Source: CAD feature listing. Evaluate the final solid. Frame: model axes, mm. Face numbers are marked on the shaded views. A direction names the side the tool comes from. Coordinates: 2 decimals unless noted, no trailing zeros. Order: outer loops, then holes, each group sorted by start corner. A loop starts at its lowest first (then second) coordinate and runs counter-clockwise, first axis right, second up.
Autodesk Inventor part; units mm, degrees
ref_plane "YZ Plane" through (0, 0, 0) normal (1, 0, 0) x (0, 1, 0)
ref_plane "XZ Plane" through (0, 0, 0) normal (0, 1, 0) x (-1, 0, 0)
ref_plane "XY Plane" through (0, 0, 0) normal (0, 0, 1) x (1, 0, 0)
sketch "Sketch1" plane through (0, 0, 0) normal (0, 1, 0) x (-1, 0, 0)
  line L0 (35, -17.5) -> (-35, -17.5)
  line L1 (-35, -17.5) -> (-35, 17.5)
  line L2 (-35, 17.5) -> (35, 17.5)
  line L3 (35, 17.5) -> (35, -17.5)
  line L4 (35, -17.5) -> (-35, 17.5) construction
  line L5 (-35, -17.5) -> (35, 17.5) construction
  point P0 (0, 0)
  dimension "d0" = 70
  dimension "d1" = 35
extrude "Extrusion1" add sketch "Sketch1" along normal blind 19.05
sketch "Sketch2" plane through (0, 19.05, 0) normal (0, 1, 0) x (1, 0, 0)
  line L0 (32.5, -15) -> (-32.5, -15)
  line L1 (-32.5, -15) -> (-32.5, 15)
  line L2 (-32.5, 15) -> (32.5, 15)
  line L3 (32.5, 15) -> (32.5, -15)
  line L4 (32.5, -15) -> (-32.5, 15) construction
  line L5 (-32.5, -15) -> (32.5, 15) construction
  point P0 (0, 0)
  dimension "d4" = 65
  dimension "d5" = 30
extrude "Extrusion2" cut sketch "Sketch2" against normal blind 1.5875
fillet "Fillet1" radius 3 4 edges at (-32.5, 18.2563, -15) (-32.5, 18.2563, 15) (32.5, 18.2563, -15) (32.5, 18.2563, 15)
sketch "Sketch3" plane through (0, 17.4625, 0) normal (0, 1, 0) x (1, 0, 0)
  arc A0 (-29.5, 15) -> (-32.5, 12) centre (-29.5, 12) ccw
  arc A1 (-32.5, -12) -> (-29.5, -15) centre (-29.5, -12) ccw
  arc A2 (29.5, -15) -> (32.5, -12) centre (29.5, -12) ccw
  arc A3 (32.5, 12) -> (29.5, 15) centre (29.5, 12) ccw
  point P0 (0, 0)
hole "Hole1" at (-29.5, 17.4625, -12) at (-29.5, 17.4625, 12) at (29.5, 17.4625, 12) at (29.5, 17.4625, -12) direction (0, -1, 0) diameter 3.175 depth 15.875
sketch "Sketch4" plane through (0, 17.4625, 0) normal (0, 1, 0) x (1, 0, 0)
  circle A0 centre (-29.5, 12) radius 1.5875 construction
  circle A1 centre (-29.5, 12) radius 3
  circle A2 centre (-29.5, -12) radius 1.5875 construction
  circle A3 centre (-29.5, -12) radius 3
  circle A4 centre (29.5, -12) radius 1.5875 construction
  arc A5 (29.5, -15) -> (32.5, -12) centre (29.5, -12) ccw
  circle A6 centre (29.5, -12) radius 3
  circle A7 centre (29.5, 12) radius 1.5875 construction
  circle A8 centre (29.5, 12) radius 3
  arc A9 (-29.5, 15) -> (-32.5, 12) centre (-29.5, 12) ccw
  arc A10 (-32.5, -12) -> (-29.5, -15) centre (-29.5, -12) ccw
  arc A11 (32.5, 12) -> (29.5, 15) centre (29.5, 12) ccw
  line L0 (-29.5, 15) -> (29.5, 15)
  line L1 (-29.5, 15) -> (29.5, 15)
  line L2 (-35, 17.5) -> (35, 17.5)
  line L3 (-32.5, -12) -> (-32.5, 12)
  line L4 (-32.5, 12) -> (-32.5, -12)
  arc A12 (-32.5, -12) -> (-29.5, -15) centre (-29.5, -12) ccw
  line L5 (-29.5, -15) -> (29.5, -15)
  line L6 (32.5, 12) -> (32.5, -12)
  line L7 (32.5, 12) -> (32.5, -12)
  point P0 (0, 0)
  point P1 (-29.5, -9)
  point P2 (-26.5, -12)
  point P3 (-29.5, 9)
  point P4 (-26.5, 12)
  point P5 (26.5, 12)
  point P6 (29.5, 9)
  point P7 (26.5, -12)
  point P8 (29.5, -9)
extrude "Extrusion3" cut sketch "Sketch4" against normal blind 14.2875 contours A1 L0 A8 L6 A6 L5 A3 L3
fillet "Fillet3" radius 3 8 edges at (-32.5, 10.3188, -12) (-29.5, 10.3188, -15) (-32.5, 10.3188, 12) (-29.5, 10.3188, 15) (29.5, 10.3188, 15) (32.5, 10.3188, 12) (29.5, 10.3188, -15) (32.5, 10.3188, -12)
sketch "Sketch6" plane through (0, 3.175, 0) normal (0, 1, 0) x (1, 0, 0)
  line L0 (-3.75, 10.5) -> (23.75, 10.5)
  line L1 (23.75, 10.5) -> (23.75, -10.5)
  line L2 (23.75, -10.5) -> (-3.75, -10.5)
  line L3 (-3.75, -10.5) -> (-3.75, 10.5)
  line L4 (-3.75, 10.5) -> (23.75, -10.5) construction
  line L5 (23.75, 10.5) -> (-3.75, -10.5) construction
  line L6 (-3.5, 14) -> (23.5, 14) construction
  line L7 (23.5, 14) -> (23.5, -14) construction
  line L8 (23.5, -14) -> (-3.5, -14) construction
  line L9 (-3.5, -14) -> (-3.5, 14) construction
  line L10 (-3.5, 14) -> (23.5, -14) construction
  line L11 (23.5, 14) -> (-3.5, -14) construction
  point P0 (0, 0)
  point P1 (10, 0)
  point P2 (10, 0)
  point P3 (10, 0)
  dimension "d22" = 27.5
  dimension "d23" = 21
  dimension "d24" = 27
  dimension "d25" = 28
  dimension "d26" = 10
extrude "Extrusion4" cut sketch "Sketch6" against normal through all
sketch "Sketch7" plane through (0, 3.175, 0) normal (0, 1, 0) x (1, 0, 0)
  line L0 (-3.75, -10.5) -> (-3.75, 10.5)
  point P0 (0, 0)
  point P1 (-18.75, 0)
  dimension "d37" = 15
hole "Hole2" at (-18.75, 3.175, 0) direction (0, -1, 0) diameter 7.5 end through all
sketch "Sketch8" plane through (0, 3.175, 0) normal (0, 1, 0) x (1, 0, 0)
  line L0 (17.5, 13.5) -> (2.5, 13.5)
  line L1 (2.5, 13.5) -> (2.5, 10.5)
  line L2 (2.5, 10.5) -> (17.5, 10.5)
  line L3 (17.5, 10.5) -> (17.5, 13.5)
  line L4 (-3.75, 10.5) -> (23.75, 10.5)
  point P0 (0, 0)
  point P1 (10, 13.5)
  point P2 (10, 10.5)
  point P3 (10, 10.5)
  dimension "d38" = 3
  dimension "d39" = 15
extrude "Extrusion5" cut sketch "Sketch8" against normal blind 1.5875
fillet "Fillet5" radius 1.5875 4 edges at (2.5, 2.3812, -13.5) (2.5, 2.3812, -10.5) (17.5, 2.3812, -13.5) (17.5, 2.3812, -10.5)
properties part number "Display Case" material "Wood (Walnut)"
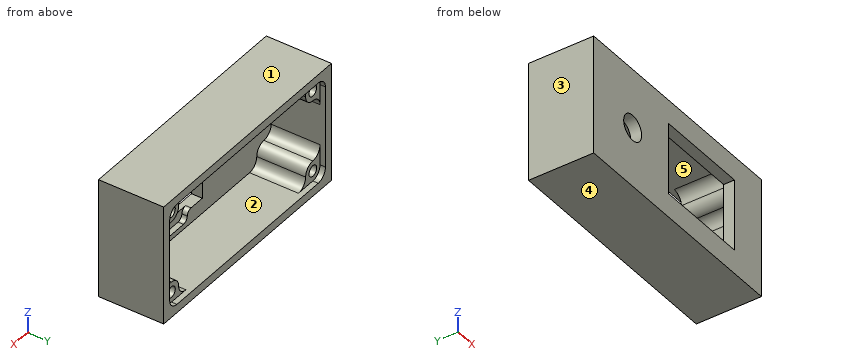
Q1. Set-up query: the marked faces 4 and 5. Return all of +Z, -Z, +X, -X, +Y, -Y with unobstructed straight access to the full face (end or side cutting, diameter ignored); none if empty.
Solutions:
face 4: -Z, +X, -X, +Y, -Y
face 5: +Y
Q2. Section query D-D on y = 2.5. Give the number of separate pieces and of enclosed holes in the cut face, plus the area to 3 significant figures.
Solutions:
separate pieces: 1
enclosed holes: 6
area: 1,750 mm2
Q3. Section query A-A on x = -21. Output: boundary loops of the cut face in (y, z) (3 decimals).
Solutions:
outline: (0, -17.5) - (19.05, -17.5) - (19.05, -15) - (3.175, -15) - (3.175, -3) - (0, -3) - close; (0, 3) - (3.175, 3) - (3.175, 15) - (19.05, 15) - (19.05, 17.5) - (0, 17.5) - close
Q4. Material intervals for line 1 along Z through (x, y) = (-29.5, 10.75); line 2 along X through (y, z) = (8.25, -12); line 3 along Z through (x, y) = (3, 6), sorted ascending.
Solutions:
line 1: z = -17.5 to -13.59, -10.41 to -9, 9 to 10.41, 13.59 to 17.5
line 2: x = -35 to -31.09, -27.91 to -26.5, 26.5 to 27.91, 31.09 to 35
line 3: z = -17.5 to -15, 15 to 17.5
Q5. Pin query (flat end, axial travel): P1, Ø2.5, axis at x = -28.5, z = 12, coming from the +Y side; P2, Ø3.5, axis at x = 29.5, z = -12, coming from the -Y side; P3, Ø2, axis at x = -3, z = -10.5, coming from the +Y side (3 decimals); P4, Ø1.5, axis at x = 13, z = -11.5, coming from the +Y side. Return the tip coordinate at first contact, or that it passes through.
Solutions:
P1: stops at y = 17.46
P2: stops at y = 0
P3: stops at y = 3.175
P4: stops at y = 1.59
Q6. Section query C-C on x = -8. Output: boundary loops of the cut face in (y, z) (3 decimals), plus the area to 4 significant figures.
Solutions:
outline: (0, -17.5) - (19.05, -17.5) - (19.05, -15) - (3.175, -15) - (3.175, 15) - (19.05, 15) - (19.05, 17.5) - (0, 17.5) - close
area: 190.5 mm2
Q7. Section query B-B on z = -5. Output: boundary loops of the cut face in (x, y) (3 decimals), plus the area to 3 significant figures.
Solutions:
outline: (-35, 0) - (-3.75, 0) - (-3.75, 3.175) - (-32.5, 3.175) - (-32.5, 19.05) - (-35, 19.05) - close; (23.75, 0) - (35, 0) - (35, 19.05) - (32.5, 19.05) - (32.5, 3.175) - (23.75, 3.175) - close
area: 214 mm2
Q8. Pull-direction query (X, two-part tool) for the marked faces 1, 2 and 3; classes: pulls with the +X half, pulls with the -X half, needs draft (parallel to the pull), parting line crosses it, or undercut.
Solutions:
face 1: needs draft
face 2: undercut
face 3: pulls with the -X half
